Input: dimensioned drawing with shaded views. Units: mm. Origin: part minimum x, y, z. A direction names the side the tool comes from. Give positions to 0.01 mm unless a question says otherwise; leave off trailing zeros. Write each loop counter-clockwise with the first axis right and the second up, starting at its lowest first coordinate (ties: lowest second). Pieces come first, ordered by that corner, then holes.
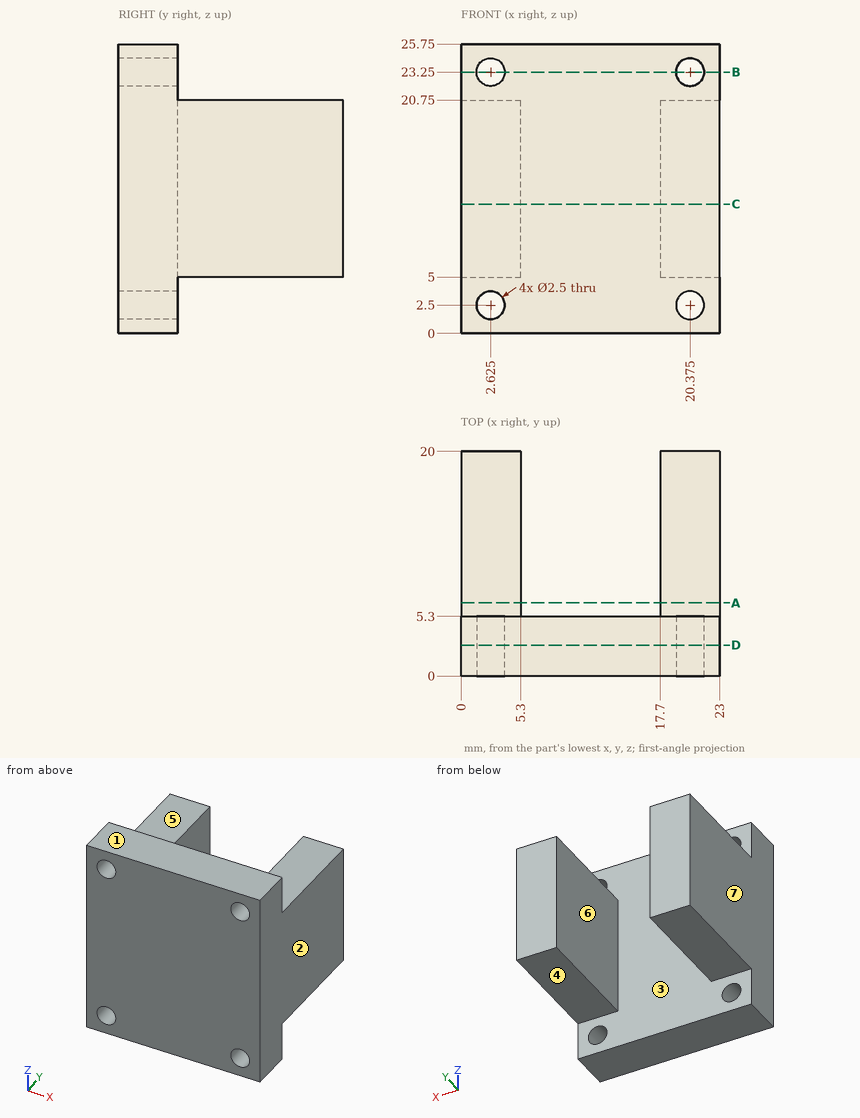
Item 1: Section C-C, the plane z = 11.5. Return the cut outline in (x, y).
Found:
outline: (0, 0) - (23, 0) - (23, 20) - (17.7, 20) - (17.7, 5.3) - (5.3, 5.3) - (5.3, 20) - (0, 20) - close
Item 2: Reachability of the marked faces 4, 5, 6 and 7 from +Z, -Z, +X, -X, +Y, -Y: full face, straight path, thin tool, end or side. Return the list, or none.
Found:
face 4: -Z, +X, -X, +Y
face 5: +Z, +X, -X, +Y
face 6: +Z, -Z, +Y
face 7: +Z, -Z, -X, +Y, -Y
Item 3: Section D-D, the plane y = 2.75. Return the cut outline in (x, z) (3 decimals), plus the area to 3 significant figures.
Found:
outline: (0, 0) - (23, 0) - (23, 25.75) - (0, 25.75) - close; hole circle Ø2.5 at (2.625, 2.5); hole circle Ø2.5 at (2.625, 23.25); hole circle Ø2.5 at (20.375, 2.5); hole circle Ø2.5 at (20.375, 23.25)
area: 573 mm2
Item 4: Pin query (flat end, axial travel): pin 1 Ø12 at (x, y) = (10, 13) entering from +Z; pin 2 Ø4 at (x, y) = (3, 12.5) entering from -Z; pin 3 Ø6 at (x, z) = (10, 18.5) entering from +Y. Return the tip coordinate at first contact, or that it passes through.
Found:
pin 1: stops at z = 20.75
pin 2: stops at z = 5
pin 3: stops at y = 5.3
Item 5: Pull-direction query (X, two-part tool) for the marked faces 1, 2 and 3; classes: +X half, -X half, draft (parallel to the pull), parting line (faces both ways), or undercut.
Found:
face 1: draft
face 2: +X half
face 3: undercut
Item 6: Section B-B, the plane z = 23.25. Return the cut outline in (x, y) (3 decimals), plus the area to 3 significant figures.
Found:
outline: (0, 0) - (1.375, 0) - (1.375, 5.3) - (0, 5.3) - close; (3.875, 0) - (19.125, 0) - (19.125, 5.3) - (3.875, 5.3) - close; (21.625, 0) - (23, 0) - (23, 5.3) - (21.625, 5.3) - close
area: 95.4 mm2
Item 7: Section A-A, the plane y = 6.5. Return the cut outline in (x, z), plus the area to 3 significant figures.
Found:
outline: (0, 5) - (5.3, 5) - (5.3, 20.75) - (0, 20.75) - close; (17.7, 5) - (23, 5) - (23, 20.75) - (17.7, 20.75) - close
area: 167 mm2
Item 8: Line query: L1, parallel to X at y = 4.05, z = 23.25 (3 decimals); L2, parallel to X at y = 5.5, z = 13; L3, parallel to Z at x = 19.75, y = 1.75. Output: solid intervals per line, ascending.
Found:
L1: x = 0 to 1.375, 3.875 to 19.125, 21.625 to 23
L2: x = 0 to 5.3, 17.7 to 23
L3: z = 0 to 1.42, 3.58 to 22.17, 24.33 to 25.75
